For this review, take the finished solid that the model builds, in its own axes (mm). Face numbers are marked on the shaded views. A direction names the side the tool comes from. Coordinates: 2 decimals unless noted, no trailing zeros. Write each loop counter-clockwise with the first axis right and the second up, starting at its lowest first coordinate (ties: lowest second). Pieces come first, ordered by that corner, then holes.
```python
from build123d import *

# Parameters (mm, degrees)
ESQUISSE1_R        = 8.5
ESQUISSE1_R_2      = 1.6
BOSS_EXTRU_1_DEPTH = 6.2
ESQUISSE2_R        = 9.7
ESQUISSE2_R_2      = 8.5
BOSS_EXTRU_2_DEPTH = 2
CHANFREIN1_SIZE    = 0.6


with BuildPart() as part:
    # Esquisse1 → Boss.-Extru.1 (new body)
    with BuildSketch(Plane.XY):
        Circle(ESQUISSE1_R)
        with Locations((-4, 2)):
            Circle(ESQUISSE1_R_2, mode=Mode.SUBTRACT)
        with Locations((4, 2)):
            Circle(ESQUISSE1_R_2, mode=Mode.SUBTRACT)
    extrude(amount=BOSS_EXTRU_1_DEPTH)

    # Esquisse2 → Boss.-Extru.2 (add)
    with BuildSketch(Plane.XY.offset(6.2)):
        Circle(ESQUISSE2_R)
        Circle(ESQUISSE2_R_2, mode=Mode.SUBTRACT)
    extrude(amount=-BOSS_EXTRU_2_DEPTH)

    # Chanfrein1
    chanfrein1_edges = [part.edges().sort_by_distance(p)[0] for p in [
        (-8.5, 0, 0),
    ]]
    chamfer(chanfrein1_edges, length=CHANFREIN1_SIZE)


solid = part.part
```
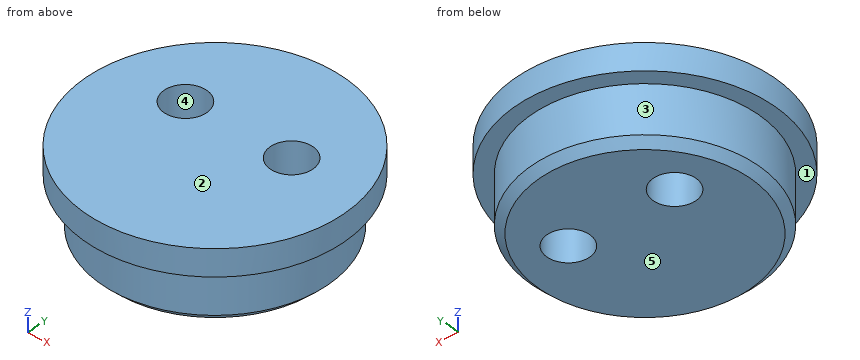
Q1. Add section C-C (y = 2). Give the number of separate pieces and of enclosed holes in the cut face, then the cut area to 3 significant figures.
Ans:
separate pieces: 3
enclosed holes: 0
area: 67.3 mm2
Q2. Draft analysis for pull direction X (two halves, no side actions). For the marked faces 3, 4 and 5, state which applies: +X half, -X half, draft (parallel to the pull), parting line (faces both ways), or undercut.
Ans:
face 3: parting line
face 4: undercut
face 5: draft
Q3. Add section D-D (z = 4.75). State the section outline as (x, y) points.
Ans:
outline: circle Ø19.4 at (0, 0); hole circle Ø3.2 at (-4, 2); hole circle Ø3.2 at (4, 2)
Q4. Tool access review of the marked faces 1 and 2: name each direction out of +Z, -Z, +X, -X, +Y, -Y from which nothing blocks a thin tool from reaching the whole face with its end or side.
Ans:
face 1: -Z
face 2: +Z, +X, -X, +Y, -Y
Q5. For probe 1 along X at (y, z) = (1.5, 3.25); probe 2 along Y at (x, z) = (-3, 5.25); probe 3 along Y at (x, z) = (-4, 3.75), list the stretches that pass through material, from the lowest coordinate up.
Ans:
probe 1: x = -8.37 to -5.52, -2.48 to 2.48, 5.52 to 8.37
probe 2: y = -9.22 to 0.75, 3.25 to 9.22
probe 3: y = -7.5 to 0.4, 3.6 to 7.5
Q6. Clearance check with flat-ended pins moving along their axes: pin 1 Ø4 at (x, y) = (4, 2) entering from +Z; pin 2 Ø2 at (y, z) = (6.5, 2) entering from +X; pin 3 Ø2 at (y, z) = (-6.5, 4.5) entering from +X; pin 4 Ø1.5 at (x, z) = (-5, 1.5) entering from -Y. State where each tip first meets the part, or that it passes through.
Ans:
pin 1: stops at z = 6.2
pin 2: stops at x = 6.48
pin 3: stops at x = 7.99
pin 4: stops at y = -7.36
Q7. Add section A-A (z = 2). State the section outline as (x, y) points.
Ans:
outline: circle Ø17 at (0, 0); hole circle Ø3.2 at (-4, 2); hole circle Ø3.2 at (4, 2)
Q8. Add section B-B (x = 0). State the section outline as (y, z) points.
Ans:
outline: (-9.7, 4.2) - (-8.5, 4.2) - (-8.5, 0.6) - (-7.9, 0) - (7.9, 0) - (8.5, 0.6) - (8.5, 4.2) - (9.7, 4.2) - (9.7, 6.2) - (-9.7, 6.2) - close
